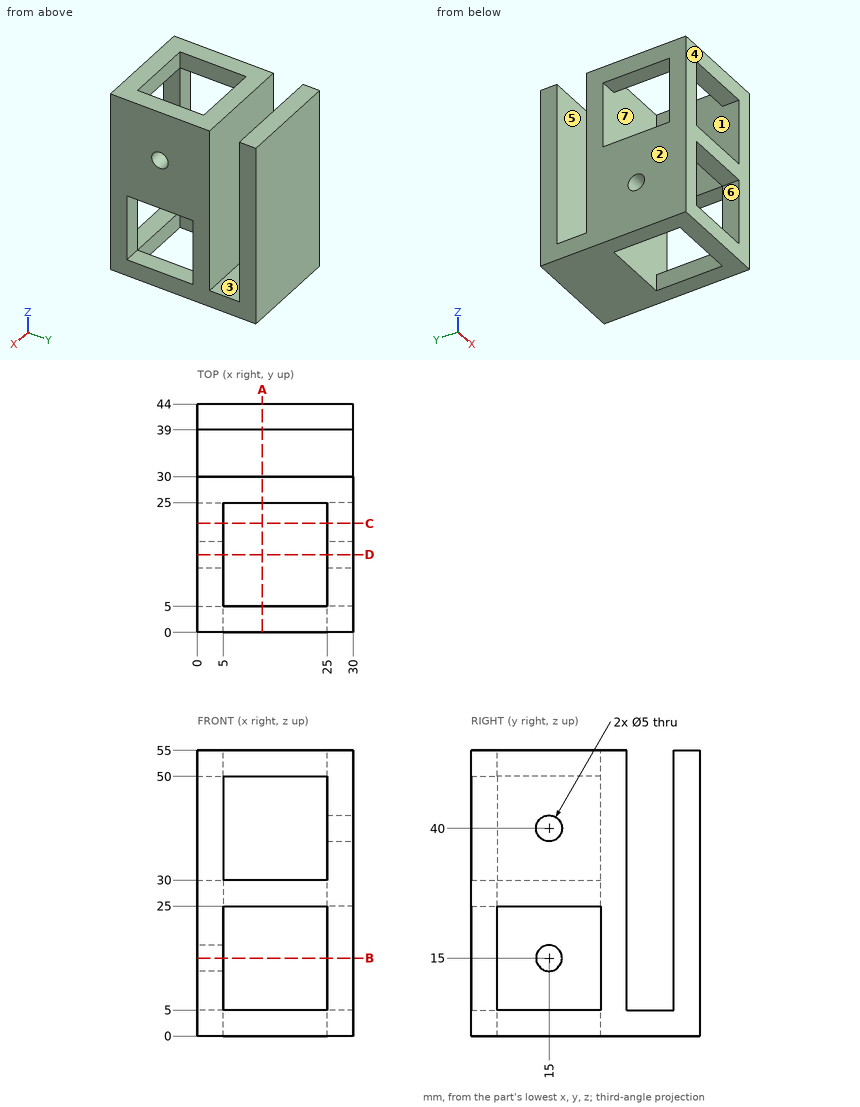
Here's the drawing with two shaded views (mm, measured from the low corner). I have some questions. A direction names the side the tool comes from. Coordinates: 2 decimals unless noted, no trailing zeros. Write each loop counter-clockwise with the first axis right and the second up, starting at its lowest first coordinate (ties: lowest second). Pieces come first, ordered by that corner, then holes.
Item 1: I want a section at B-B on z = 15. Write out the boundary of the cut face in (x, y), and give its area (3 significant figures).
Item 2: Will these pins go through, and if not, where does the flat tip stop? pin 1 (8 mm diameter, centred on y = 15, z = 15, fed in from +X); pin 2 (4.5 mm diameter, centred on x = 22, y = 35, fed in from +Z); pin 3 (7.5 mm diameter, centred on y = 13.5, z = 38.5, fed in from -X); pin 4 (3 mm diameter, centred on x = 23, y = 22, fed in from +Z).
Item 3: I want a section at D-D on y = 15. Write out the boundary of the cut face in (x, z), and give its area (3 significant figures).
Item 4: If we mould it in two halves opening along Y, with no side actions, what happens to the marked faces 1, 2, 3 and 4? For each: +Y half, -Y half, draft (parallel to the pull), parting line (faces both ways), or undercut.
Item 5: On a 3-axis mill with a long thin cutter (end or side, diameter ignored), from which of +Z, -Z, +X, -X, +Y, -Y can I reach the whole of each face in a straight line? I mean the marked faces 5, 6 and 7. Say none if no direction works.
Item 6: I want a section at A-A on x = 12.5. Write out the boundary of the cut face in (y, z), and give its area (3 significant figures).
Item 7: If I drill on line 1 (Y direction, x = 26, z = 20.5); line 2 (Z direction, x = 11.75, y = 4.5); line 3 (Y direction, x = 28.1, z = 40), over which ranges is the centre line in solid material (lowest first)?
Item 8: I want a section at C-C on y = 21. Write out the boundary of the cut face in (x, z).
Findings below:
1. outline: (0, 0) - (5, 0) - (5, 12.5) - (0, 12.5) - close; (0, 17.5) - (5, 17.5) - (5, 25) - (30, 25) - (30, 30) - (0, 30) - close; (0, 39) - (30, 39) - (30, 44) - (0, 44) - close; (25, 0) - (30, 0) - (30, 5) - (25, 5) - close
1. area: 425 mm2
2. pin 1: stops at x = 5
2. pin 2: stops at z = 5
2. pin 3: stops at x = 25
2. pin 4: passes through
3. outline: (0, 0) - (5, 0) - (5, 12.5) - (0, 12.5) - close; (0, 17.5) - (5, 17.5) - (5, 30) - (0, 30) - close; (0, 50) - (5, 50) - (5, 55) - (0, 55) - close; (25, 0) - (30, 0) - (30, 5) - (25, 5) - close; (25, 25) - (30, 25) - (30, 37.5) - (25, 37.5) - close; (25, 42.5) - (30, 42.5) - (30, 55) - (25, 55) - close
3. area: 300 mm2
4. face 1: undercut
4. face 2: draft
4. face 3: undercut
4. face 4: -Y half
5. face 5: +Z, +X, -X
5. face 6: -Y
5. face 7: none
6. outline: (0, 0) - (5, 0) - (5, 5) - (0, 5) - close; (0, 25) - (5, 25) - (5, 30) - (0, 30) - close; (0, 50) - (5, 50) - (5, 55) - (0, 55) - close; (25, 0) - (44, 0) - (44, 55) - (39, 55) - (39, 5) - (30, 5) - (30, 55) - (25, 55) - close
6. area: 670 mm2
7. line 1: y = 0 to 5, 25 to 30, 39 to 44
7. line 2: z = 0 to 5, 25 to 30, 50 to 55
7. line 3: y = 0 to 12.5, 17.5 to 30, 39 to 44
8. outline: (0, 0) - (5, 0) - (5, 30) - (0, 30) - close; (0, 50) - (5, 50) - (5, 55) - (0, 55) - close; (25, 0) - (30, 0) - (30, 5) - (25, 5) - close; (25, 25) - (30, 25) - (30, 55) - (25, 55) - close
